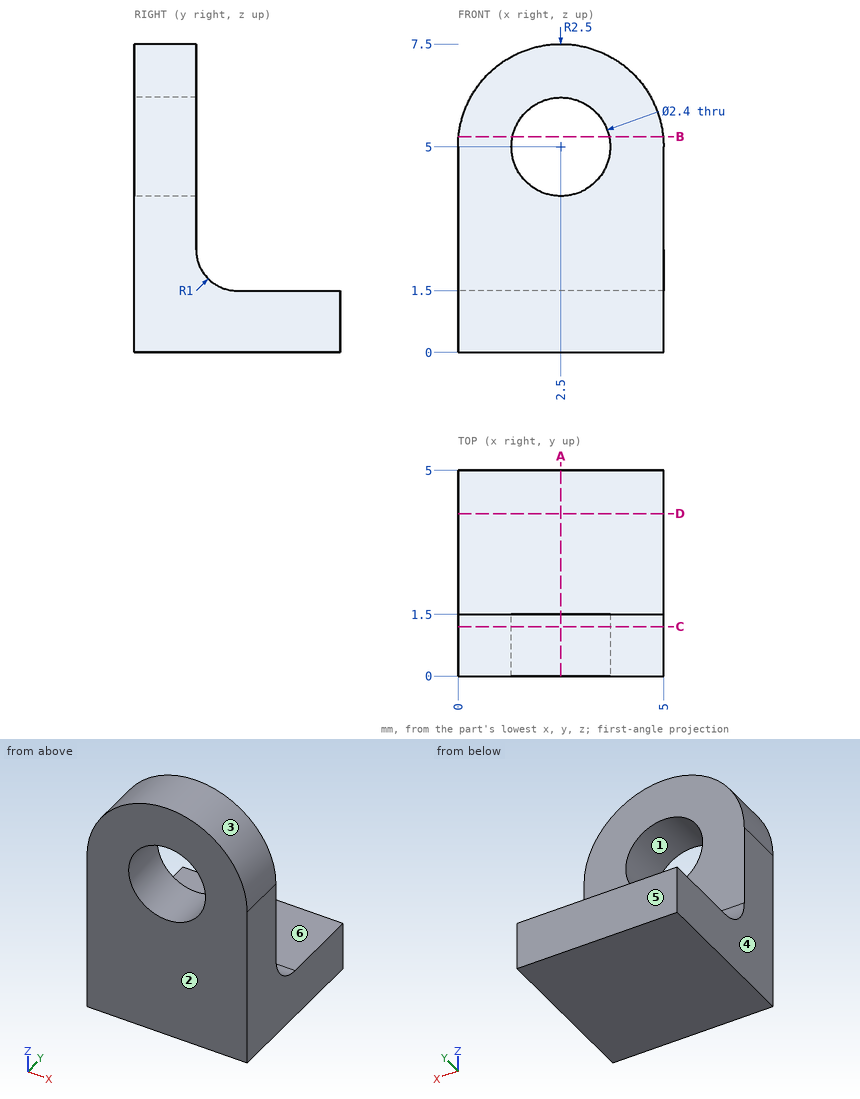
Could you check a few things on this drawing? It's one solid part, dimensions in mm from its lowest x, y, z. A direction names the side the tool comes from. Coordinates: 2 decimals unless noted, no trailing zeros. Order: outer loops, then holes, each group sorted by start corner. A loop starts at its lowest first (then second) coordinate and runs counter-clockwise, first axis right, second up. Notation, with made-up numbers: M 34,37 L 62,37 A14 cw 62,42 Z; hole C 75,26 d2. An arc over 180 degrees is marked long. Use one line per item in the form item = value. Start each with the question number.
1. Suppose I cut it at A-A on x = 2.5. Write out the boundary of the cut face in (y, z).
2. Please list where these lines run through material, in increasing order: line 1 (Z direction, x = 2.5, y = 1.15); line 2 (X direction, y = 0.55, z = 4.75); line 3 (Y direction, x = 1.3, z = 3.5).
3. Suppose I cut it at D-D on y = 3.95. Write out the boundary of the cut face in (x, z).
4. Suppose I cut it at B-B on z = 5.25. Write out the boundary of the cut face in (x, y).
5. For pin 1 (1 mm diameter, centred on x = 1.5, y = 4, fed in from +Z); pin 2 (1.4 mm diameter, centred on x = 2.5, z = 5, fed in from -Y), each with a flat end and sliding along its axis, tell me the tip position at first contact or that it passes through.
6. Suppose I cut it at C-C on y = 1.2. Write out the boundary of the cut face in (x, z).
7. On a 3-axis mill with a long thin cutter (end or side, diameter ignored), from which of +Z, -Z, +X, -X, +Y, -Y can I reach the whole of each face in a straight line? I mean the marked faces 5 and 6. Say none if no direction works.
8. We'd pull the mould along X, two halves only. Please class the marked faces 1, 2, 3 and 4: +X half, -X half, draft (parallel to the pull), parting line (faces both ways), or undercut.
Geometry says:
q1.outline = M 0,0 L 5,0 L 5,1.5 L 2.5,1.5 A1 cw 1.5,2.5 L 1.5,3.8 L 0,3.8 Z; M 0,6.2 L 1.5,6.2 L 1.5,7.5 L 0,7.5 Z
q2.line_1 = 0 to 3.8, 6.2 to 7.5
q2.line_2 = 0 to 1.33, 3.67 to 5
q2.line_3 = 0 to 1.5
q3.outline = M 0,0 L 5,0 L 5,1.5 L 0,1.5 Z
q4.outline = M 0.01,0 L 1.33,0 L 1.33,1.5 L 0.01,1.5 Z; M 3.67,0 L 4.99,0 L 4.99,1.5 L 3.67,1.5 Z
q5.pin_1 = 1.5
q5.pin_2 = through
q6.outline = M 0,0 L 5,0 L 5,5 A2.5 ccw 0,5 Z; hole C 2.5,5 d2.4
q7.face_5 = +Z, -Z, +X, -X, +Y
q7.face_6 = +Z, +X, -X, +Y
q8.face_1 = undercut
q8.face_2 = draft
q8.face_3 = parting line
q8.face_4 = -X half
